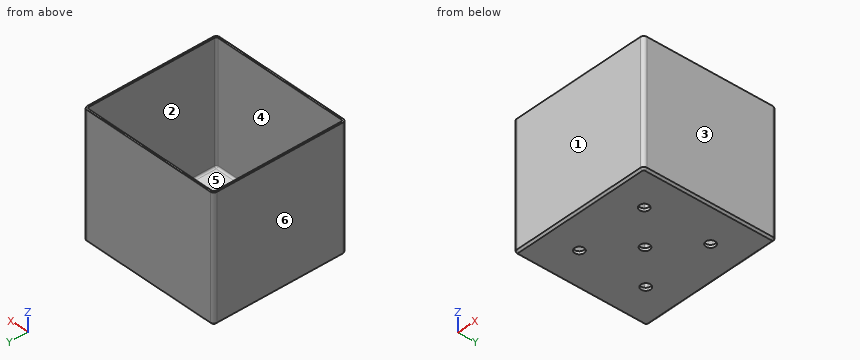
```python
from build123d import *

# Parameters (mm, degrees)
SKETCH_W        = 150
SKETCH_H        = 140
PAD_DEPTH       = 130
SKETCH001_W     = 146.4
SKETCH001_H     = 136.4
POCKET_DEPTH    = 127
SKETCH002_R     = 5
POCKET001_DEPTH = 130.001
FILLET_R        = 2
FILLET001_R     = 3.6
CHAMFER_SIZE    = 2


with BuildPart() as part:
    # Sketch → Pad (new body)
    with BuildSketch(Plane.XY):
        Rectangle(SKETCH_W, SKETCH_H)
    extrude(amount=PAD_DEPTH)

    # Sketch001 (on DatumPlane) → Pocket (cut)
    with BuildSketch(Plane.XY.offset(130)):
        Rectangle(SKETCH001_W, SKETCH001_H)
    extrude(amount=-POCKET_DEPTH, mode=Mode.SUBTRACT)

    # Sketch002 → Pocket001 (cut, through all)
    with BuildSketch(Plane.XY):
        with Locations((-37.5, 35)):
            Circle(SKETCH002_R)
        with Locations((37.5, 35)):
            Circle(SKETCH002_R)
        with Locations((37.5, -35)):
            Circle(SKETCH002_R)
        with Locations((-37.5, -35)):
            Circle(SKETCH002_R)
        Circle(SKETCH002_R)
    extrude(amount=POCKET001_DEPTH, mode=Mode.SUBTRACT)

    # Fillet
    fillet_edges = [part.edges().sort_by_distance(p)[0] for p in [
        (-73.2, 68.2, 66.5),
        (0, 68.2, 3),
        (-73.2, 0, 3),
        (-73.2, -68.2, 66.5),
        (0, -68.2, 3),
        (73.2, -68.2, 66.5),
        (73.2, 0, 3),
        (73.2, 68.2, 66.5),
    ]]
    fillet(fillet_edges, radius=FILLET_R)

    # Fillet001
    fillet001_edges = [part.edges().sort_by_distance(p)[0] for p in [
        (-75, -70, 65),
        (75, -70, 65),
        (75, 70, 65),
        (-75, 70, 65),
    ]]
    fillet(fillet001_edges, radius=FILLET001_R)

    # Chamfer
    chamfer_edges = [part.edges().sort_by_distance(p)[0] for p in [
        (0, 70, 0),
    ]]
    chamfer(chamfer_edges, length=CHAMFER_SIZE)


solid = part.part
```
Input: part model. Units: mm. Frame: model coordinates. Face numbers are marked on the shaded views. A direction names the side the tool comes from. Give positions to 0.01 mm unless a question says otherwise; leave off trailing zeros. Order: outer loops, then holes, each group sorted by start corner. A loop starts at its lowest first (then second) coordinate and runs counter-clockwise, first axis right, second up.
1. Cut plane A-A (x = 37.5). Return loops of the section in (y, z).
Computed:
outline: (-70, 2) - (-68, 0) - (-40, 0) - (-40, 3) - (-66.2, 3) arc R2 cw to (-68.2, 5) - (-68.2, 130) - (-70, 130) - close; (-30, 0) - (30, 0) - (30, 3) - (-30, 3) - close; (40, 0) - (68, 0) - (70, 2) - (70, 130) - (68.2, 130) - (68.2, 5) arc R2 cw to (66.2, 3) - (40, 3) - close
2. Draft query along Y for the marked faces 1, 2, 3 and 4. Return one class per face: released by +Y, released by -Y, zero draft, split by the parting line, or undercut.
Computed:
face 1: released by -Y
face 2: undercut
face 3: zero draft
face 4: undercut
3. Line query: probe 1 along X at (y, z) = (35, 2.05); probe 2 along Y at (x, z) = (-37.5, 2.2); probe 3 along Y at (x, z) = (-6, 106). Output: solid intervals per line, ascending.
Computed:
probe 1: x = -75 to -42.5, -32.5 to 32.5, 42.5 to 75
probe 2: y = -70 to -40, -30 to 30, 40 to 70
probe 3: y = -70 to -68.2, 68.2 to 70
4. Set-up query: the marked faces 5 and 6. Return all of +Z, -Z, +X, -X, +Y, -Y with unobstructed straight access to the full face (end or side cutting, diameter ignored); none if empty.
Computed:
face 5: +Z
face 6: +Z, -Z, -X, +Y, -Y
5. Cut plane C-C (x = 0). Return loops of the section in (y, z).
Computed:
outline: (-70, 2) - (-68, 0) - (-5, 0) - (-5, 3) - (-66.2, 3) arc R2 cw to (-68.2, 5) - (-68.2, 130) - (-70, 130) - close; (5, 0) - (68, 0) - (70, 2) - (70, 130) - (68.2, 130) - (68.2, 5) arc R2 cw to (66.2, 3) - (5, 3) - close
6. Cut plane D-D (z = 13.5). Return loops of the section in (x, y).
Computed:
outline: (-75, -66.4) arc R3.6 ccw to (-71.4, -70) - (71.4, -70) arc R3.6 ccw to (75, -66.4) - (75, 66.4) arc R3.6 ccw to (71.4, 70) - (-71.4, 70) arc R3.6 ccw to (-75, 66.4) - close; hole (-73.2, -66.2) arc R2 ccw to (-71.2, -68.2) - (71.2, -68.2) arc R2 ccw to (73.2, -66.2) - (73.2, 66.2) arc R2 ccw to (71.2, 68.2) - (-71.2, 68.2) arc R2 ccw to (-73.2, 66.2) - close
7. Pin query (flat end, axial travel): pin 1 Ø13 at (x, y) = (-37.5, 35) entering from +Z. Return the tip coordinate at first contact, or that it passes through.
Computed:
pin 1: stops at z = 3
8. Cut plane B-B (y = 0). Return loops of the section in (x, z), and give its area (3 significant figures).
Computed:
outline: (-75, 2) - (-73, 0) - (-5, 0) - (-5, 3) - (-71.2, 3) arc R2 cw to (-73.2, 5) - (-73.2, 130) - (-75, 130) - close; (5, 0) - (73, 0) - (75, 2) - (75, 130) - (73.2, 130) - (73.2, 5) arc R2 cw to (71.2, 3) - (5, 3) - close
area: 875 mm2
